from build123d import *

# Parameters (mm, degrees)
F0_R     = 40
F1_DEPTH = 25
F2_R     = 1.6
F3_DEPTH = 85.4176260163
F4_R     = 1.6
F5_DEPTH = 85.4176260163


with BuildPart() as f1:
    # F0 (on Top) → F1 (new body)
    with BuildSketch(Plane.XY):
        with BuildLine():
            Line((42.7083130081, -5), (42.7083130081, 5))
            ThreePointArc((42.7083130081, 5), (30.405591591, 30.405591591), (5, 42.7083130081))
            Line((5, 42.7083130081), (-5, 42.7083130081))
            ThreePointArc((-5, 42.7083130081), (-30.405591591, 30.405591591), (-42.7083130081, 5))
            Line((-42.7083130081, 5), (-42.7083130081, -5))
            ThreePointArc((-42.7083130081, -5), (-30.405591591, -30.405591591), (-5, -42.7083130081))
            Line((-5, -42.7083130081), (5, -42.7083130081))
            ThreePointArc((5, -42.7083130081), (30.405591591, -30.405591591), (42.7083130081, -5))
        make_face()
        Circle(F0_R, mode=Mode.SUBTRACT)
    extrude(amount=F1_DEPTH)

    # F2 (on face) → F3 (cut, through all)
    with BuildSketch(Plane.YZ.offset(42.7083130081)):
        with Locations((0, 17.5)):
            Circle(F2_R)
        with Locations((0, 7.5)):
            Circle(F2_R)
    extrude(amount=-F3_DEPTH, mode=Mode.SUBTRACT)

    # F4 (on face) → F5 (cut, through all)
    with BuildSketch(Plane.XZ.offset(42.7083130081)):
        with Locations((0, 17.5)):
            Circle(F4_R)
        with Locations((0, 7.5)):
            Circle(F4_R)
    extrude(amount=-F5_DEPTH, mode=Mode.SUBTRACT)


solid = f1.part
Geometry: final body of the model. Coordinates: model frame, mm. Coordinates: 2 decimals unless noted, no trailing zeros. Loops run counter-clockwise (first coordinate to the right, second up) from the corner with the lowest first, then second, coordinate; pieces in that order, holes last. Notation, with made-up numbers: M 5,-22 L 23,-22 A18 cw 23,9 Z; hole C 78.25,14 d8. An arc over 180 degrees is marked long. One line per item, written item: value. Start each with the question number.
1) Pin query (flat end, axial travel): P1, Ø6, axis at x = 18.5, z = 11.5, coming from the -Y side; P2, Ø1, axis at x = 9.5, z = 12, coming from the -Y side; P3, Ø4, axis at y = 18.5, z = 6.5, coming from the -X side. Return the tip coordinate at first contact, or that it passes through.
2) Cut plane A-A (x = 0). Return loops of the section in (y, z), then the cut area to 3 significant figures.
3) Cut plane D-D (y = 34). Return loops of the section in (x, z), then the cut area to 3 significant figures.
4) Material intervals for L1, parallel to Z at x = 0, y = -41; L2, parallel to Y at x = 0, z = 12.75; L3, parallel to X at y = 23, z = 4, sorted ascending. Write a range as from..to.
5) Cut plane B-B (z = 17.5). Return loops of the section in (x, y).
6) Draft query along Y for faces 1 (the cylindrical face through (-41.32, -0.35, 5.94)), 2 (the flat face through (42.708, 0, 12)), 3 (the cylindrical face through (-30.69, -30.12, 12.32)). Return one class per face: released by +Y, released by -Y, zero draft, split by the parting line, or undercut.
Evaluation:
1. P1: y = -40.11
1. P2: y = -42.05
1. P3: x = -39.71
2. outline: M -42.71,0 L -40,0 L -40,5.9 L -42.71,5.9 Z; M -42.71,9.1 L -40,9.1 L -40,15.9 L -42.71,15.9 Z; M -42.71,19.1 L -40,19.1 L -40,25 L -42.71,25 Z; M 40,0 L 42.71,0 L 42.71,5.9 L 40,5.9 Z; M 40,9.1 L 42.71,9.1 L 42.71,15.9 L 40,15.9 Z; M 40,19.1 L 42.71,19.1 L 42.71,25 L 40,25 Z
2. area: 101 mm^2
3. outline: M -26.32,0 L -21.07,0 L -21.07,25 L -26.32,25 Z; M 21.07,0 L 26.32,0 L 26.32,25 L 21.07,25 Z
3. area: 263 mm^2
4. L1: 0..5.9, 9.1..15.9, 19.1..25
4. L2: -42.71..-40, 40..42.71
4. L3: -36.33..-32.73, 32.73..36.33
5. outline: M -42.71,-5 A43 ccw -5,-42.71 L -1.6,-42.71 L -1.6,-39.97 A40 cw -39.97,-1.6 L -42.71,-1.6 Z; M -42.71,1.6 L -39.97,1.6 A40 cw -1.6,39.97 L -1.6,42.71 L -5,42.71 A43 ccw -42.71,5 Z; M 1.6,-42.71 L 5,-42.71 A43 ccw 42.71,-5 L 42.71,-1.6 L 39.97,-1.6 A40 cw 1.6,-39.97 Z; M 1.6,39.97 A40 cw 39.97,1.6 L 42.71,1.6 L 42.71,5 A43 ccw 5,42.71 L 1.6,42.71 Z
6. face 1: undercut
6. face 2: zero draft
6. face 3: released by -Y
